```python
from build123d import *

# Parameters (mm, degrees)
F0_R     = 45
F0_R_2   = 7.075
F1_DEPTH = 8
F2_R     = 17.5
F2_R_2   = 11.5
F3_DEPTH = 30


# Not quite as in the source:
# - a fillet or chamfer that OpenCascade refuses, or shapes differently, is made with other operations: its cross-section is extruded or revolved along the edge and cut away or added


with BuildPart() as f1:
    # F0 (on Top) → F1 (new body)
    with BuildSketch(Plane.XY):
        Circle(F0_R)
        Circle(F0_R_2, mode=Mode.SUBTRACT)
    extrude(amount=F1_DEPTH)

    # F2 (on face) → F3 (join)
    with BuildSketch(Plane.XY.offset(8)):
        Circle(F2_R)
        Circle(F2_R_2, mode=Mode.SUBTRACT)
    extrude(amount=F3_DEPTH)

    # F4: fillet of radius 6 on 4 edges, made by hand

    # F4_s1 → F4_t2 (revolve)
    with BuildSketch(Plane.XZ):
        with BuildLine():
            ThreePointArc((23.5009656854, 7.9996), (19.2573593129, 9.7573593129), (17.4996, 14.0009656854))
            Line((17.4996, 14.0009656854), (16.8994634315, 14.0009656854))
            ThreePointArc((16.8994634315, 14.0009656854), (16.8998634315, 11.0004828427), (16.8998634315, 8))
            Line((16.8998634315, 8), (17.5, 7.3998634315))
            ThreePointArc((17.5, 7.3998634315), (20.5004828427, 7.3998634315), (23.5009656854, 7.3994634315))
            Line((23.5009656854, 7.3994634315), (23.5009656854, 7.9996))
        make_face()
    revolve(axis=Axis((0, 0, 8), (0, 0, 1)))

    # F4_s3 → F4_t4 (revolve)
    with BuildSketch(Plane.XZ):
        with BuildLine():
            ThreePointArc((7.0751050475, 7.9996140401), (10.2674180504, 10.1463065699), (11.5004, 13.7903299833))
            Line((11.5004, 13.7903299833), (12.1005365685, 13.7903299833))
            ThreePointArc((12.1005365685, 13.7903299833), (12.1001365685, 10.8951649917), (12.1001365685, 8))
            Line((12.1001365685, 8), (11.5, 7.3998634315))
            ThreePointArc((11.5, 7.3998634315), (9.2875525237, 7.3998634315), (7.2327121208, 7.4205424458))
            Line((7.2327121208, 7.4205424458), (7.0751050475, 7.9996140401))
        make_face()
    revolve(axis=Axis((0, 0, 8), (0, 0, 1)))

    # F4_s5 → F4_t6 (revolve, cut)
    with BuildSketch(Plane.XZ):
        with BuildLine():
            ThreePointArc((45.0004, 1.9990343146), (43.2426406871, 6.2426406871), (38.9990343146, 8.0004))
            Line((38.9990343146, 8.0004), (38.9990343146, 8.6005365685))
            ThreePointArc((38.9990343146, 8.6005365685), (41.9995171573, 8.6001365685), (45, 8.6001365685))
            Line((45, 8.6001365685), (45.6001365685, 8))
            ThreePointArc((45.6001365685, 8), (45.6001365685, 4.9995171573), (45.6005365685, 1.9990343146))
            Line((45.6005365685, 1.9990343146), (45.0004, 1.9990343146))
        make_face()
    revolve(axis=Axis((0, 0, 8), (0, 0, 1)), mode=Mode.SUBTRACT)

    # F4_s7 → F4_t8 (revolve, cut)
    with BuildSketch(Plane.XZ):
        with BuildLine():
            ThreePointArc((17.5004, 31.9990343923), (15.7429821175, 36.242299307), (11.5000000644, 38.0004))
            Line((11.5000000644, 38.0004), (11.5000966393, 38.6005365608))
            ThreePointArc((11.5000966393, 38.6005365608), (14.5000000322, 38.6001365685), (17.5, 38.6001365685))
            Line((17.5, 38.6001365685), (18.1001365685, 38))
            ThreePointArc((18.1001365685, 38), (18.1001365685, 34.9995171961), (18.1005365685, 31.9990343923))
            Line((18.1005365685, 31.9990343923), (17.5004, 31.9990343923))
        make_face()
    revolve(axis=Axis((0, 0, 38), (0, 0, 1)), mode=Mode.SUBTRACT)


solid = f1.part
```
Verification items for the finished model (mm, model axes). Coordinates: 2 decimals unless noted, no trailing zeros. Loops run counter-clockwise (first coordinate to the right, second up) from the corner with the lowest first, then second, coordinate; pieces in that order, holes last. Notation, with made-up numbers: (53, 66.25) -> (80, 66.25) arc R36 cw to (80, 105.25) -> close; hole circle Ø3 at (77, 76). An arc over 180 degrees is marked (long way). Answer in a Markdown table with one row per item.
1) Depth check by flat-ended pin: P1, Ø5, axis at x = 11, z = 25.5, coming from the +Y side; P2, Ø8, axis at x = -9, y = 31, coming from the -Z side; P3, Ø10, axis at x = 26, y = -4.5, coming from the +Z side; P4, Ø1, axis at y = -15, z = 24.5, coming from the +X side. Enter the tip coordinate at first touch or a pass-through.
The answers:
| item | result |
|---|---|
| P1 | stops at y = 15.3 |
| P2 | stops at z = 0 |
| P3 | stops at z = 8.38 |
| P4 | stops at x = 9.8 |
2) Section check A-A (z = 25.5). Record the cut outline in (x, y), and give its area (3 significant figures).
The answers:
| item | result |
|---|---|
| outline | circle Ø35 at (0, 0); hole circle Ø23 at (0, 0) |
| area | 547 mm2 |
3) Scan lines: line 1 along X through (y, z) = (0, 24.75); line 2 along Y through (x, z) = (0, 2.25) (3 decimals). Record each from-to range of solid material in increasing order. Write a range as from..to.
The answers:
| item | result |
|---|---|
| line 1 | x = -17.5..-11.5, 11.5..17.5 |
| line 2 | y = -44.995..-7.075, 7.075..44.995 |
4) Section check B-B (z = 34). Record the cut outline in (x, y).
The answers:
| item | result |
|---|---|
| outline | circle Ø34.31 at (0, 0); hole circle Ø23 at (0, 0) |
5) Draft check along Y on faces 1 (the face through (20.765, -39.923, 1.02)), 2 (the face through (-1, -9, 0)), 3 (the face through (3.26, -6.28, 3.94)). Enter one of: released by +Y, released by -Y, zero draft, split by the parting line, or undercut.
The answers:
| item | result |
|---|---|
| face 1 | split by the parting line |
| face 2 | zero draft |
| face 3 | undercut |
